from build123d import *

# Parameters (mm, degrees)
SKETCH2_W           = 11
SKETCH2_H           = 22
BOSS_EXTRUDE1_DEPTH = 22
SKETCH3_W           = 11
SKETCH3_H           = 4.5
BOSS_EXTRUDE2_DEPTH = 2
SKETCH4_R           = 5.5
BOSS_EXTRUDE3_DEPTH = 4
SKETCH5_R           = 3
BOSS_EXTRUDE4_DEPTH = 4.5


with BuildPart() as part:
    # Sketch2 → Boss-Extrude1 (new body)
    with BuildSketch(Plane(origin=(0, 0, 0), x_dir=(1, 0, 0), z_dir=(0, 1, 0))):
        Rectangle(SKETCH2_W, SKETCH2_H)
    extrude(amount=BOSS_EXTRUDE1_DEPTH)

    # Sketch3 → Boss-Extrude2 (add)
    with BuildSketch(Plane(origin=(0, 15, 0), x_dir=(1, 0, 0), z_dir=(0, 1, 0))):
        with Locations((0, 13.25)):
            Rectangle(SKETCH3_W, SKETCH3_H)
        with Locations((0, -13.25)):
            Rectangle(SKETCH3_W, SKETCH3_H)
    extrude(amount=BOSS_EXTRUDE2_DEPTH)

    # Sketch4 → Boss-Extrude3 (add)
    with BuildSketch(Plane(origin=(0, 22, 0), x_dir=(1, 0, 0), z_dir=(0, 1, 0))):
        with Locations((0, 5.5)):
            Circle(SKETCH4_R)
    extrude(amount=BOSS_EXTRUDE3_DEPTH)

    # Sketch5 → Boss-Extrude4 (add)
    with BuildSketch(Plane(origin=(0, 26, 0), x_dir=(1, 0, 0), z_dir=(0, 1, 0))):
        with Locations((0, 5.5)):
            Circle(SKETCH5_R)
    extrude(amount=BOSS_EXTRUDE4_DEPTH)


solid = part.part
Geometry: final body of the model. Coordinates: model frame, mm. A direction names the side the tool comes from. Coordinates: 2 decimals unless noted, no trailing zeros. Write each loop counter-clockwise with the first axis right and the second up, starting at its lowest first coordinate (ties: lowest second). Pieces come first, ordered by that corner, then holes. Notation, with made-up numbers: (-32, 88.25) - (-8, 88.25) arc R22 cw to (-8, 127.25) - close; hole circle Ø11 at (-28, -24.5). An arc over 180 degrees is marked (long way). Return JSON: item names as keys, results as strings.
Item 1: Line query: L1, parallel to Y at x = 0.75, z = -2; L2, parallel to Y at x = 2.75, z = -0.5; L3, parallel to Z at x = -2.5, y = 5. Output: solid intervals per line, ascending.
Completed:
{"L1": "y = 0 to 26", "L2": "y = 0 to 22", "L3": "z = -11 to 11"}
Item 2: Reachability of faces 1 (the face through (0, 17, 13)), 2 (the face through (-4, 22, -10)), 3 (the face through (-1.19, 23.97, -0.13)) from +Z, -Z, +X, -X, +Y, -Y: full face, straight path, thin tool, end or side. Return the list, or none.
Completed:
{"face 1": "+Z, +X, -X, +Y", "face 2": "-Z, -X, +Y", "face 3": "+Y"}
Item 3: Pin query (flat end, axial travel): pin 1 Ø3.5 at (x, y) = (-0.5, 8.5) entering from -Z; pin 2 Ø1.5 at (x, z) = (-3.5, -10) entering from +Y; pin 3 Ø3 at (x, y) = (-0.5, 12) entering from +Z; pin 4 Ø6 at (x, z) = (-3.5, -9) entering from +Y. Return the tip coordinate at first contact, or that it passes through.
Completed:
{"pin 1": "stops at z = -11", "pin 2": "stops at y = 26", "pin 3": "stops at z = 11", "pin 4": "stops at y = 30.5"}
Item 4: Section query C-C (y = 17.5). Output: boundary loops of the cut face in (x, z), and give its area (3 significant figures).
Completed:
{"outline": "(-5.5, -11) - (5.5, -11) - (5.5, 11) - (-5.5, 11) - close", "area": "242 mm2"}
Item 5: Section query B-B (z = -1.5). Output: boundary loops of the cut face in (x, y), and give its area (3 significant figures).
Completed:
{"outline": "(-5.5, 0) - (5.5, 0) - (5.5, 22) - (3.77, 22) - (3.77, 26) - (-3.77, 26) - (-3.77, 22) - (-5.5, 22) - close", "area": "272 mm2"}
Item 6: Section query A-A (x = 1.75). Output: boundary loops of the cut face in (y, z), and give its area (3 significant figures).
Completed:
{"outline": "(0, -11) - (15, -11) - (15, -15.5) - (17, -15.5) - (17, -11) - (22, -11) - (22, -10.71) - (26, -10.71) - (26, -7.94) - (30.5, -7.94) - (30.5, -3.06) - (26, -3.06) - (26, -0.29) - (22, -0.29) - (22, 11) - (17, 11) - (17, 15.5) - (15, 15.5) - (15, 11) - (0, 11) - close", "area": "566 mm2"}
Item 7: Section query D-D (x = 4). Output: boundary loops of the cut face in (y, z), and give its area (3 significant figures).
Completed:
{"outline": "(0, -11) - (15, -11) - (15, -15.5) - (17, -15.5) - (17, -11) - (22, -11) - (22, -9.27) - (26, -9.27) - (26, -1.73) - (22, -1.73) - (22, 11) - (17, 11) - (17, 15.5) - (15, 15.5) - (15, 11) - (0, 11) - close", "area": "532 mm2"}
